```python
from build123d import *

# Parameters (mm, degrees)
F0_W     = 54
F0_H     = 54
F1_DEPTH = 54
F2_W     = 19
F2_H     = 8
F3_DEPTH = 10
F4_W     = 2.25403
F4_H     = 10.847496
F5_DEPTH = 25
F6_R     = 2.804292
F7_DEPTH = 3


with BuildPart() as f1:
    # F0 (on Top) → F1 (new body)
    with BuildSketch(Plane.XY):
        Rectangle(F0_W, F0_H)
    extrude(amount=F1_DEPTH)

    # F2 (on face) → F3 (cut)
    with BuildSketch(Plane.XY.offset(54)):
        Rectangle(F2_W, F2_H)
    extrude(amount=-F3_DEPTH, mode=Mode.SUBTRACT)

    # F4 (on face) → F5 (join)
    with BuildSketch(Plane(origin=(0, 0, 0), x_dir=(1, 0, 0), z_dir=(0, 0, -1))):
        with Locations((-15.003354, 0)):
            Rectangle(F4_W, F4_H)
    extrude(amount=F5_DEPTH)

    # F6 (on face) → F7 (cut)
    with BuildSketch(Plane(origin=(-16.130369, 0, 0), x_dir=(0, -1, 0), z_dir=(-1, 0, 0))):
        with Locations((0, -19.652281)):
            Circle(F6_R)
    extrude(amount=-F7_DEPTH, mode=Mode.SUBTRACT)

    # F8: F1 across plane


with BuildPart() as f1_1:
    add(f1.part)
    add(f1.part.mirror(Plane.YZ))


solid = f1_1.part
```
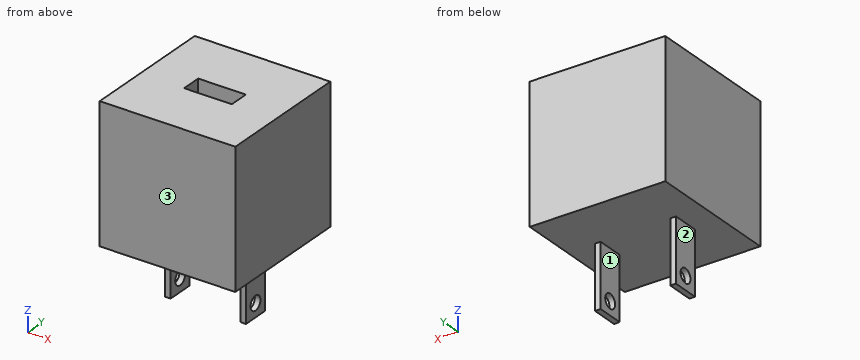
Build history of the part. All positions in model axes, mm. Face numbers are marked on the shaded views. A direction names the side the tool comes from. Coordinates: 2 decimals unless noted, no trailing zeros. Write each loop counter-clockwise with the first axis right and the second up, starting at its lowest first coordinate (ties: lowest second). Pieces come first, ordered by that corner, then holes.
1. Drop flat-ended pins along their axis: pin 1 (12 mm diameter, centred on y = -0.5, z = -15, fed in from +X); pin 2 (4 mm diameter, centred on x = 0.5, y = 13.5, fed in from -Z); pin 3 (1.1 mm diameter, centred on x = 15, z = -18.5, fed in from +Y). Give the stop position or say it passes through.
Answer block:
pin 1: stops at x = 16.13
pin 2: stops at z = 0
pin 3: stops at y = 5.42
2. Band-saw the part on B-B, the plane y = 0. Give the cut face in (x, z), and give its area (3 significant figures).
Answer block:
outline: (-27, 0) - (-16.13, 0) - (-16.13, -16.85) - (-13.88, -16.85) - (-13.88, 0) - (13.88, 0) - (13.88, -16.85) - (16.13, -16.85) - (16.13, 0) - (27, 0) - (27, 54) - (9.5, 54) - (9.5, 44) - (-9.5, 44) - (-9.5, 54) - (-27, 54) - close; (-16.13, -25) - (-13.88, -25) - (-13.88, -22.46) - (-16.13, -22.46) - close; (13.88, -25) - (16.13, -25) - (16.13, -22.46) - (13.88, -22.46) - close
area: 2,810 mm2
3. 3-axis set-ups, long thin cutter, end or side, ignore diameter. For the marked faces 1, 2 and 3: which of +Z, -Z, +X, -X, +Y, -Y reach the whole face in a straight line?
Answer block:
face 1: -Z, +Y, -Y
face 2: -Z, -X, +Y, -Y
face 3: +Z, -Z, +X, -X, -Y
4. Band-saw the part on A-A, the plane z = -15. Give the cut face in (x, y), and give its area (3 significant figures).
Answer block:
outline: (-16.13, -5.42) - (-13.88, -5.42) - (-13.88, 5.42) - (-16.13, 5.42) - close; (13.88, -5.42) - (16.13, -5.42) - (16.13, 5.42) - (13.88, 5.42) - close
area: 48.9 mm2
5. Band-saw the part on C-C, the plane x = 6.5. Give the cut face in (y, z).
Answer block:
outline: (-27, 0) - (27, 0) - (27, 54) - (4, 54) - (4, 44) - (-4, 44) - (-4, 54) - (-27, 54) - close
6. Drill centre lines: probe 1 along Z at (x, y) = (-15.25, 0); probe 2 along X at (y, z) = (2, 51); probe 3 along X at (y, z) = (-3, -7). Where is each one in solid material? Low to high.
Answer block:
probe 1: z = -25 to -22.46, -16.85 to 54
probe 2: x = -27 to -9.5, 9.5 to 27
probe 3: x = -16.13 to -13.88, 13.88 to 16.13
7. Band-saw the part on D-D, the plane x = -15. Give the cut face in (y, z).
Answer block:
outline: (-27, 0) - (-5.42, 0) - (-5.42, -25) - (5.42, -25) - (5.42, 0) - (27, 0) - (27, 54) - (-27, 54) - close; hole circle Ø5.61 at (0, -19.65)
